```python
from build123d import *

# Parameters (mm, degrees)
SKETCH011_W     = 78
SKETCH011_H     = 89.2
PAD007_DEPTH    = 3
POCKET004_DEPTH = 5
CHAMFER006_SIZE = 2
SKETCH013_W     = 15
SKETCH013_H     = 73
PAD008_DEPTH    = 3
CHAMFER007_SIZE = 2
SKETCH014_W     = 150
SKETCH014_H     = 69.2
PAD009_DEPTH    = 3
FILLET002_R     = 5


with BuildPart() as part:
    # Sketch011 (on XZ_Plane007 of Origin014) → Pad007 (new body)
    with BuildSketch(Plane.XZ):
        with Locations((39, 0)):
            Rectangle(SKETCH011_W, SKETCH011_H)
    extrude(amount=PAD007_DEPTH)

    # Sketch012 (on XZ_Plane007 of Origin014) → Pocket004 (cut)
    with BuildSketch(Plane.XZ):
        with BuildLine():
            ThreePointArc((74, 39.8), (75.7, 41.5), (74, 43.2))
            Line((74, 43.2), (70, 43.2))
            ThreePointArc((70, 43.2), (68.3, 41.5), (70, 39.8))
            Line((74, 39.8), (70, 39.8))
        make_face()
    pocket004 = extrude(amount=POCKET004_DEPTH, mode=Mode.SUBTRACT)

    # Mirrored004: Pocket004 across XY
    add(pocket004.mirror(Plane.XY), mode=Mode.SUBTRACT)

    # Mirrored005: part across YZ


with BuildPart() as part_1:
    add(part.part)
    add(part.part.mirror(Plane.YZ))

    # Chamfer006
    chamfer006_edges = [part_1.edges().sort_by_distance(p)[0] for p in [
        (78, -1.5, -44.6),
        (78, -1.5, 44.6),
        (-78, -1.5, -44.6),
        (-78, -1.5, 44.6),
    ]]
    chamfer(chamfer006_edges, length=CHAMFER006_SIZE)

    # Sketch013 (on XZ_Plane007 of Origin014) → Pad008 (join)
    with BuildSketch(Plane.XZ):
        with Locations((85.5, 0)):
            Rectangle(SKETCH013_W, SKETCH013_H)
    extrude(amount=PAD008_DEPTH)

    # Chamfer007
    chamfer007_edges = [part_1.edges().sort_by_distance(p)[0] for p in [
        (93, -1.5, -36.5),
        (93, -1.5, 36.5),
    ]]
    chamfer(chamfer007_edges, length=CHAMFER007_SIZE)

    # Sketch014 (on Face5 of Chamfer007) → Pad009 (join)
    with BuildSketch(Plane.XZ.offset(3)):
        Rectangle(SKETCH014_W, SKETCH014_H)
    extrude(amount=PAD009_DEPTH)

    # Fillet002
    fillet002_edges = [part_1.edges().sort_by_distance(p)[0] for p in [
        (75, -4.5, 34.6),
        (75, -4.5, -34.6),
        (-75, -4.5, 34.6),
        (-75, -4.5, -34.6),
    ]]
    fillet(fillet002_edges, radius=FILLET002_R)


solid = part_1.part
```
Could you check a few things on this model? Use its own coordinates, in mm. A direction names the side the tool comes from. Give positions to 0.01 mm unless a question says otherwise; leave off trailing zeros. Loops run counter-clockwise (first coordinate to the right, second up) from the corner with the lowest first, then second, coordinate; pieces in that order, holes last. Notation, with made-up numbers: (-23, 8) -> (27, 8) arc R13 cw to (27, 26) -> close; hole circle Ø4 at (34.5, -6). An arc over 180 degrees is marked (long way). Put each result on its own line as item: value.
(1) Please list where these lines run through material, in increasing order: probe 1 along Z at (x, y) = (-1, -3.4); probe 2 along Y at (x, z) = (-61, 38); probe 3 along X at (y, z) = (-0.85, -37.5). Write a range as [from, to].
Computed:
probe 1: [-34.6, 34.6]
probe 2: [-3, 0]
probe 3: [-78, 78]
(2) Thinking about a two-plate mould opening in Z: for faces 5 (the face through (73.57, -4.52, -33.1)), 6 (the face through (75.7, -1.5, -41.5)), 7 (the face through (78, -1, 40)), which applies, pulls with the +Z half, pulls with the -Z half, needs draft (parallel to the pull), parting line crosses it, or undercut?
Computed:
face 5: pulls with the -Z half
face 6: undercut
face 7: needs draft
(3) I'm going to push flat-ended pins straight in: pin 1 Ø0.9 at (y, z) = (-4.5, 1) entering from +X; pin 2 Ø1.5 at (x, y) = (83.5, -1.5) entering from -Z; pin 3 Ø0.9 at (y, z) = (-5, 1) entering from -X. Where does each tip first touch, or does it pass through?
Computed:
pin 1: x = 75
pin 2: z = -36.5
pin 3: x = -75
(4) Imagine slicing it at C-C on x = -65.5. Write out the boundary of the cut face in (y, z).
Computed:
outline: (-6, -34.6) -> (-3, -34.6) -> (-3, -44.6) -> (0, -44.6) -> (0, 44.6) -> (-3, 44.6) -> (-3, 34.6) -> (-6, 34.6) -> close
(5) Imagine slicing it at B-B on z = -4.5. Write out the boundary of the cut face in (x, y).
Computed:
outline: (-78, -3) -> (-75, -3) -> (-75, -6) -> (75, -6) -> (75, -3) -> (93, -3) -> (93, 0) -> (-78, 0) -> close
(6) Imagine slicing it at A-A on y = -2.05. State how many separate pieces and enclosed holes the cut face has, plus the area to 3 significant figures.
Computed:
separate pieces: 1
enclosed holes: 4
area: 14,900 mm^2
(7) For faces 1 (the face through (-75.7, -1.5, 41.5)), 2 (the face through (84, -1, -36.5)), 3 (the face through (-1, -4, 34.6)), 4 (the face through (-75, -4, 0)), which set-ups out of +Z, -Z, +X, -X, +Y, -Y let a thin tool reach every point of the face, with its end or its side?
Computed:
face 1: +Y, -Y
face 2: -Z, +X, +Y, -Y
face 3: +Z, +X, -X, -Y
face 4: +Z, -Z, -X, -Y
